Design review of the part built by this model. Coordinates are the model's own, in mm. A direction names the side the tool comes from. Give positions to 0.01 mm unless a question says otherwise; leave off trailing zeros. Loops run counter-clockwise (first coordinate to the right, second up) from the corner with the lowest first, then second, coordinate; pieces in that order, holes last. Notation, with made-up numbers: (88.5, 56) -> (115.5, 56) arc R34 cw to (115.5, 87) -> close; hole circle Ø2 at (31, 61). An arc over 180 degrees is marked (long way). Use CSV: the item, a comma, the result in double quotes. Start each with the question number.
Item 1: We need section D-D (z = 4.5). State the section outline as (x, y) points, plus the area to 3 significant figures.
Item 2: Clearance check with flat-ended pins moving along their axes: pin 1 (7.5 mm diameter, centred on x = 2, z = 0.5, fed in from -Y); pin 2 (3 mm diameter, centred on x = -2, z = -2.5, fed in from -Y). State where each tip first meets the part, or that it passes through.
Item 3: Wall thickness on line 1 along X through (y, z) = (1.2, -1); line 2 along Z through (x, y) = (7, 2.8); line 3 along Z through (x, y) = (3, 4.55): over which ranges is each line inside the solid? List them lowest first. Write a range as from..to.
Item 4: We need section A-A (z = 0). State the section outline as (x, y) points, plus the area to 3 significant figures.
Item 5: We need section C-C (y = 3.45). State the section outline as (x, z) points.
Item 6: The part is to be moulded in two halves that separate along Z. For faces 3 (the face through (9.638, 2.958, 6.268)), 4 (the face through (18, 3, 0)), 5 (the face through (-4.88, 4.99, -1.08)), say which applies: +Z half, -Z half, draft (parallel to the pull), parting line (faces both ways), or undercut.
Item 7: For faces 1 (the face through (-9.638, 2.958, -6.268)), 2 (the face through (5, 4, 2)), list the 3-axis set-ups (+Z, -Z, +X, -X, +Y, -Y) from which the entire face can be reached by the end or side of a thin tool; tool diameter is ignored.
Item 8: We need section B-B (x = 0). State the section outline as (y, z) points, plus the area to 3 significant figures.
from build123d import *

# Parameters (mm, degrees)
SKETCH1_R           = 2
SKETCH1_R_2         = 9.6
SKETCH1_R_3         = 7.6
BOSS_EXTRUDE1_DEPTH = 4
SKETCH2_R           = 5
SKETCH2_R_2         = 2
BOSS_EXTRUDE2_DEPTH = 2


with BuildPart() as part:
    # Sketch1 → Boss-Extrude1 (new body)
    # profile 1 of 3: a face of its own
    with BuildSketch(Plane(origin=(0, 0, 0), x_dir=(1, 0, 0), z_dir=(0, 1, 0))):
        with BuildLine():
            ThreePointArc((-3.84, -8.798545334), (-9.6, 0), (-3.84, 8.798545334))
            Line((-3.84, 8.798545334), (-15.6, 3.666060556))
            ThreePointArc((-15.6, 3.666060556), (-18, 0), (-15.6, -3.666060556))
            Line((-15.6, -3.666060556), (-3.84, -8.798545334))
        make_face()
        with Locations(Location((-14, 0, 0), (0, 0, 270))):
            Circle(SKETCH1_R, mode=Mode.SUBTRACT)
    # profile 2 of 3: a face of its own
    with BuildSketch(Plane(origin=(0, 0, 0), x_dir=(1, 0, 0), z_dir=(0, 1, 0))):
        Circle(SKETCH1_R_2)
        with Locations(Location((0, 0, 0), (0, 0, 270))):
            Circle(SKETCH1_R_3, mode=Mode.SUBTRACT)
    # profile 3 of 3: a face of its own
    with BuildSketch(Plane(origin=(0, 0, 0), x_dir=(1, 0, 0), z_dir=(0, 1, 0))):
        with BuildLine():
            Line((15.6, 3.666060556), (3.84, 8.798545334))
            ThreePointArc((3.84, 8.798545334), (8.031936255, 5.258136552), (9.6, 0))
            ThreePointArc((9.6, 0), (8.031936255, -5.258136552), (3.84, -8.798545334))
            Line((3.84, -8.798545334), (15.6, -3.666060556))
            ThreePointArc((15.6, -3.666060556), (18, 0), (15.6, 3.666060556))
        make_face()
        with Locations(Location((14, 0, 0), (0, 0, 270))):
            Circle(SKETCH1_R, mode=Mode.SUBTRACT)
    extrude(amount=BOSS_EXTRUDE1_DEPTH)

    # Sketch2 → Boss-Extrude2 (add)
    with BuildSketch(Plane(origin=(0, 4, 0), x_dir=(1, 0, 0), z_dir=(0, 1, 0))):
        with BuildLine():
            Line((-3.84, 8.798545334), (-15.6, 3.666060556))
            ThreePointArc((-15.6, 3.666060556), (-18, 0), (-15.6, -3.666060556))
            Line((-15.6, -3.666060556), (-3.84, -8.798545334))
            ThreePointArc((-3.84, -8.798545334), (0, -9.6), (3.84, -8.798545334))
            Line((3.84, -8.798545334), (15.6, -3.666060556))
            ThreePointArc((15.6, -3.666060556), (18, 0), (15.6, 3.666060556))
            Line((15.6, 3.666060556), (3.84, 8.798545334))
            ThreePointArc((3.84, 8.798545334), (0, 9.6), (-3.84, 8.798545334))
        make_face()
        with Locations(Location((0, 0, 0), (0, 0, 270))):
            Circle(SKETCH2_R, mode=Mode.SUBTRACT)
        with Locations(Location((-14, 0, 0), (0, 0, 270))):
            Circle(SKETCH2_R_2, mode=Mode.SUBTRACT)
        with Locations(Location((14, 0, 0), (0, 0, 270))):
            Circle(SKETCH2_R_2, mode=Mode.SUBTRACT)
    extrude(amount=BOSS_EXTRUDE2_DEPTH)


solid = part.part
Results found:
1,outline,"(-13.69, 0) -> (-6.12, 0) -> (-6.12, 4) -> (-2.18, 4) -> (-2.18, 6) -> (-13.69, 6) -> close; (2.18, 4) -> (6.12, 4) -> (6.12, 0) -> (13.69, 0) -> (13.69, 6) -> (2.18, 6) -> close"
1,area,"107 mm²"
2,pin 1,"y = 4"
2,pin 2,"through"
3,line 1,"-17.87..-15.73, -12.27..-7.53, 7.53..12.27, 15.73..17.87"
3,line 2,"-7.42..-2.96, 2.96..7.42"
3,line 3,"-9.12..-4, 4..9.12"
4,outline,"(-18, 0) -> (-16, 0) -> (-16, 6) -> (-18, 6) -> close; (-12, 0) -> (-7.6, 0) -> (-7.6, 4) -> (-5, 4) -> (-5, 6) -> (-12, 6) -> close; (5, 4) -> (7.6, 4) -> (7.6, 0) -> (12, 0) -> (12, 6) -> (5, 6) -> close; (16, 0) -> (18, 0) -> (18, 6) -> (16, 6) -> close"
4,area,"87.2 mm²"
5,outline,"(-15.6, -3.67) -> (-3.84, -8.8) arc R9.6 ccw to (3.84, -8.8) -> (15.6, -3.67) arc R4 ccw to (15.6, 3.67) -> (3.84, 8.8) arc R9.6 ccw to (-3.84, 8.8) -> (-15.6, 3.67) arc R4 ccw to start; hole circle Ø4 at (-14, 0); hole circle Ø15.2 at (0, 0); hole circle Ø4 at (14, 0)"
6,face 3,"+Z half"
6,face 4,"parting line"
6,face 5,"undercut"
7,face 1,"-Z, -X, +Y, -Y"
7,face 2,"-Y"
8,outline,"(0, -9.6) -> (6, -9.6) -> (6, -5) -> (4, -5) -> (4, -7.6) -> (0, -7.6) -> close; (0, 7.6) -> (4, 7.6) -> (4, 5) -> (6, 5) -> (6, 9.6) -> (0, 9.6) -> close"
8,area,"34.4 mm²"
